Here's how the part is built. I have some questions about the finished solid (model axes, mm). Face numbers are marked on the shaded views. A direction names the side the tool comes from. Coordinates: 2 decimals unless noted, no trailing zeros. Write each loop counter-clockwise with the first axis right and the second up, starting at its lowest first coordinate (ties: lowest second). Pieces come first, ordered by that corner, then holes.
Item 1: I'm going to push flat-ended pins straight in: pin 1 Ø17 at (y, z) = (53.35, -30.8) entering from -X; pin 2 Ø12 at (x, z) = (81.5, 6.5) entering from -Y; pin 3 Ø2 at (x, y) = (13.5, 8.5) entering from +Z. Where does each tip first touch, or does it pass through?
Item 2: If we section it at C-C (x = 25.5): Please give me the cut outline in (y, z).
Item 3: If we section it at A-A (z = 0): Please give me the cut outline in (x, y), then the cut area to 3 significant figures.
Item 4: For the marked faces 4 and 5, which set-ups out of +Z, -Z, +X, -X, +Y, -Y let a thin tool reach every point of the face, with its end or its side?
Item 5: If we section it at D-D (x = 8): Please give me the cut outline in (y, z), then the cut area to 3 significant figures.
Item 6: If I drill on line 1 (Z direction, x = 25, y = 0); line 2 (X direction, y = -11, z = 42); line 3 (Z direction, x = 40, y = -7.5), over which ranges is the centre line in solid material (lowest first)?
Item 7: If we section it at B-B (y = 0): Please give me the cut outline in (x, z), then the cut area to 3 significant figures.
Item 8: We'd pull the mould along Y, two halves only. Please class the marked faces 1, 2 and 3: +Y half, -Y half, draft (parallel to the pull), parting line (faces both ways), or undercut.
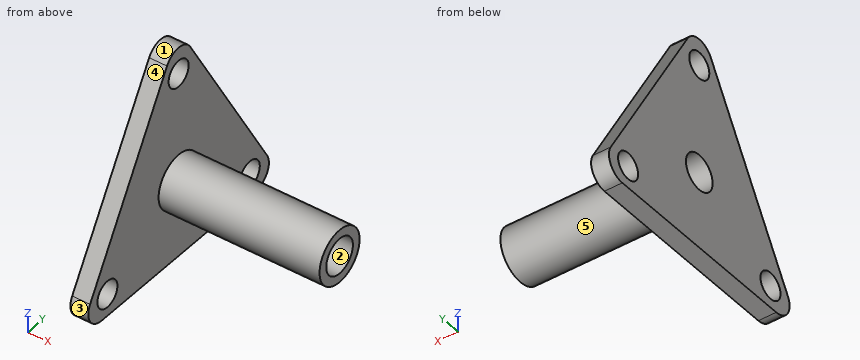
from build123d import *

# Parameters (mm, degrees)
F0_R     = 15
F0_R_2   = 10
F1_DEPTH = 100
F3_DEPTH = 10
F4_R     = 10
F5_R     = 7.5
F5_R_2   = 10
F6_DEPTH = 100.001


with BuildPart() as f1:
    # F0 (on Right) → F1 (new body)
    with BuildSketch(Plane.YZ):
        Circle(F0_R)
        Circle(F0_R_2, mode=Mode.SUBTRACT)
    extrude(amount=F1_DEPTH)

    # F2 (on Right) → F3 (join)
    with BuildSketch(Plane.YZ):
        Polygon((0, 86.60254), (-75, -43.30127), (75, -43.30127), align=None)
    extrude(amount=F3_DEPTH)

    # F4
    f4_edges = [f1.edges().sort_by_distance(p)[0] for p in [
        (5, 0, 86.60254),
        (5, 75, -43.30127),
        (5, -75, -43.30127),
    ]]
    fillet(f4_edges, radius=F4_R)

    # F5 (on Right) → F6 (cut, through all)
    with BuildSketch(Plane.YZ):
        with Locations((0, 61.60254)):
            Circle(F5_R)
        with Locations((53.349365, -30.80127)):
            Circle(F5_R)
        with Locations((-53.349365, -30.80127)):
            Circle(F5_R)
        Circle(F5_R_2)
    extrude(amount=F6_DEPTH, mode=Mode.SUBTRACT)


solid = f1.part
Answer list:
1. pin 1: stops at x = 0
1. pin 2: stops at y = -14.99
1. pin 3: stops at z = 12.99
2. outline: circle Ø30 at (0, 0); hole circle Ø20 at (0, 0)
3. outline: (0, -50) - (10, -50) - (10, -15) - (100, -15) - (100, -10) - (0, -10) - close; (0, 10) - (100, 10) - (100, 15) - (10, 15) - (10, 50) - (0, 50) - close
3. area: 1,700 mm2
4. face 4: +Z, +X, -X, -Y
4. face 5: +X
5. outline: (-66.34, -28.3) arc R10 ccw to (-57.68, -43.3) - (57.68, -43.3) arc R10 ccw to (66.34, -28.3) - (8.66, 71.6) arc R10 ccw to (-8.66, 71.6) - close; hole circle Ø15 at (-53.35, -30.8); hole circle Ø20 at (0, 0); hole circle Ø15 at (0, 61.6); hole circle Ø15 at (53.35, -30.8)
5. area: 8,690 mm2
6. line 1: z = -15 to -10, 10 to 15
6. line 2: x = 0 to 10
6. line 3: z = -12.99 to -6.61, 6.61 to 12.99
7. outline: (0, -43.3) - (10, -43.3) - (10, -15) - (100, -15) - (100, -10) - (0, -10) - close; (0, 10) - (100, 10) - (100, 15) - (10, 15) - (10, 54.1) - (0, 54.1) - close; (0, 69.1) - (10, 69.1) - (10, 76.6) - (0, 76.6) - close
7. area: 1,750 mm2
8. face 1: parting line
8. face 2: undercut
8. face 3: -Y half
